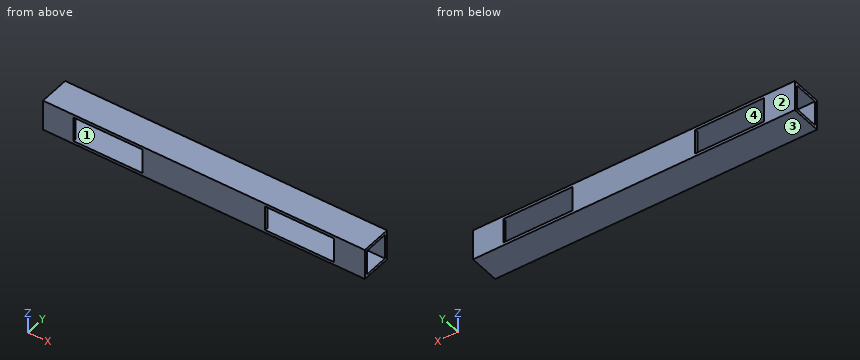
```python
from build123d import *

# Parameters (mm, degrees)
F0_W     = 1066.8
F0_H     = 101.6
F1_DEPTH = 50.8
F2_W     = 82.55
F2_H     = 82.55
F3_DEPTH = 1066.801
F4_W     = 228.6
F4_H     = 82.55
F5_DEPTH = 101.601


with BuildPart() as f1:
    # F0 (on Top) → F1 (new body, symmetric)
    with BuildSketch(Plane.XY):
        Rectangle(F0_W, F0_H)
    extrude(amount=F1_DEPTH, both=True)

    # F2 (on face) → F3 (cut, through all)
    with BuildSketch(Plane.YZ.offset(533.4)):
        Rectangle(F2_W, F2_H)
    extrude(amount=-F3_DEPTH, mode=Mode.SUBTRACT)

    # F4 (on face) → F5 (cut, through all)
    with BuildSketch(Plane.XZ.offset(50.8)):
        with Locations((-317.5, 0)):
            Rectangle(F4_W, F4_H)
        with Locations((317.5, 0)):
            Rectangle(F4_W, F4_H)
    extrude(amount=-F5_DEPTH, mode=Mode.SUBTRACT)


solid = f1.part
```
Work out the finished part from the listing and answer in its coordinate system (mm). Face numbers are marked on the shaded views. Give positions to 0.01 mm unless a question says otherwise; leave off trailing zeros. Order: outer loops, then holes, each group sorted by start corner. A loop starts at its lowest first (then second) coordinate and runs counter-clockwise, first axis right, second up. Notation, with made-up numbers: M -32,-31 L 11,-31 A13 ccw 11,-27 Z; hole C 16.25,59 d3. An arc over 180 degrees is marked long. Return JSON: item names as keys, results as strings.
1) Section B-B, the plane y = -23 is taken. Write down the section's boundary in (x, z) (3 decimals).
Resolved:
{"outline": "M -533.4,-50.8 L 533.4,-50.8 L 533.4,-41.275 L -533.4,-41.275 Z; M -533.4,41.275 L 533.4,41.275 L 533.4,50.8 L -533.4,50.8 Z"}
2) For a pull along Z with two mould halves and no side action, classify the marked faces 1, 2, 3 and 4 as +Z half, -Z half, draft (parallel to the pull), parting line (faces both ways), or undercut.
Resolved:
{"face 1": "undercut", "face 2": "draft", "face 3": "-Z half", "face 4": "undercut"}
3) Section D-D, the plane x = -454.5 is taken. Write down the section's boundary in (y, z) (3 decimals), plus the area to 3 significant figures.
Resolved:
{"outline": "M -50.8,-50.8 L 50.8,-50.8 L 50.8,50.8 L -50.8,50.8 Z; hole M -41.275,-41.275 L 41.275,-41.275 L 41.275,41.275 L -41.275,41.275 Z", "area": "3,510 mm^2"}
4) Section A-A, the plane z = 16 is taken. Write down the section's boundary in (x, y) (3 decimals), plus the area to 3 significant figures.
Resolved:
{"outline": "M -533.4,-50.8 L -431.8,-50.8 L -431.8,-41.275 L -533.4,-41.275 Z; M -533.4,41.275 L -431.8,41.275 L -431.8,50.8 L -533.4,50.8 Z; M -203.2,-50.8 L 203.2,-50.8 L 203.2,-41.275 L -203.2,-41.275 Z; M -203.2,41.275 L 203.2,41.275 L 203.2,50.8 L -203.2,50.8 Z; M 431.8,-50.8 L 533.4,-50.8 L 533.4,-41.275 L 431.8,-41.275 Z; M 431.8,41.275 L 533.4,41.275 L 533.4,50.8 L 431.8,50.8 Z", "area": "11,600 mm^2"}
5) Section C-C, the plane x = 215.5 is taken. Write down the section's boundary in (y, z) (3 decimals), plus the area to 3 significant figures.
Resolved:
{"outline": "M -50.8,-50.8 L 50.8,-50.8 L 50.8,-41.275 L -50.8,-41.275 Z; M -50.8,41.275 L 50.8,41.275 L 50.8,50.8 L -50.8,50.8 Z", "area": "1,940 mm^2"}
6) Straight lines are drawn through the part: line 1 along X through (y, z) = (44, -34); line 2 along Z through (x, y) = (-301, -30) (3 decimals). For each, find the intervals that lie inside material, in ascending order. Write a range as [from, to].
Resolved:
{"line 1": "[-533.4, -431.8], [-203.2, 203.2], [431.8, 533.4]", "line 2": "[-50.8, -41.275], [41.275, 50.8]"}
7) This flat-tipped pin is pushed along its axis until it touches: pin 1 (12 mm diameter, centred on y = -39, z = 2.5, fed in from +X). Where does it stop, or does it pass through?
Resolved:
{"pin 1": "x = 533.4"}
